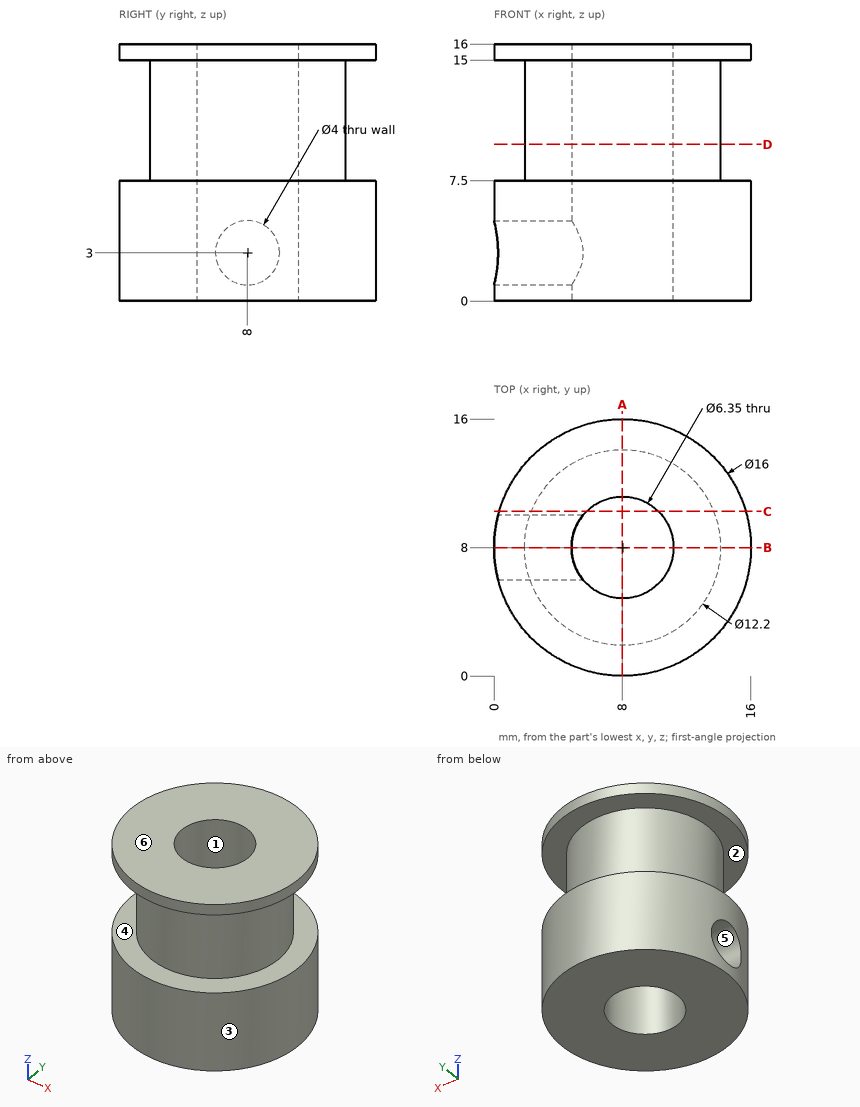
For this review, use the dimensioned drawing (mm, ordinates from the lowest corner) and the shaded views. A direction names the side the tool comes from. Coordinates: 2 decimals unless noted, no trailing zeros. Order: outer loops, then holes, each group sorted by start corner. A loop starts at its lowest first (then second) coordinate and runs counter-clockwise, first axis right, second up. Notation, with made-up numbers: (22.25, 29.25) - (33.25, 29.25) arc R19 cw to (33.25, 58.25) - close; hole circle Ø3 at (-21.5, 46.25). An arc over 180 degrees is marked (long way). Answer as a JSON object with one key per item and string values. Group by question number.
1. Clearance check with flat-ended pins moving along their axes: P1, Ø2, axis at x = 12.5, z = 9, coming from the +Y side; P2, Ø1.5, axis at x = 6, z = 5, coming from the -Y side; P3, Ø1.5, axis at y = 10.5, z = 12, coming from the -X side. State where each tip first meets the part, or that it passes through.
2. We need section D-D on z = 9.75. State the section outline as (x, y) points (3 decimals).
3. We need section A-A on x = 8. State the section outline as (y, z) points (3 decimals).
4. The part is to be moulded in two halves that separate along X. For the marked faces 1, 2 and 3, say which applies: pulls with the +X half, pulls with the -X half, needs draft (parallel to the pull), parting line crosses it, or undercut.
5. We need section B-B on y = 8. State the section outline as (x, z) points (3 decimals).
6. For probe 1 along Z at (x, y) = (14.5, 5.25); probe 2 along Y at (x, z) = (8, 4) (3 decimals); probe 3 along Y at (x, z) = (8, 10.75) (3 decimals), list the stretches that pass through material, from the lowest coordinate up.
7. For the marked faces 4, 5 and 6, list the 3-axis set-ups (+Z, -Z, +X, -X, +Y, -Y) from which the entire face can be reached by the end or side of a thin tool; tool diameter is ignored.
8. We need section C-C on y = 10.25. State the section outline as (x, z) points, then the cut area to 3 significant figures.
Final values:
{
 "1": {"P1": "y = 13", "P2": "y = 0.1", "P3": "x = 2.16"},
 "2": {"outline": "circle Ø12.2 at (8, 8); hole circle Ø6.35 at (8, 8)"},
 "3": {"outline": "(0, 0) - (4.825, 0) - (4.825, 16) - (0, 16) - (0, 15) - (1.9, 15) - (1.9, 7.5) - (0, 7.5) - close; (11.175, 0) - (16, 0) - (16, 7.5) - (14.1, 7.5) - (14.1, 15) - (16, 15) - (16, 16) - (11.175, 16) - close"},
 "4": {"face 1": "undercut", "face 2": "needs draft", "face 3": "parting line crosses it"},
 "5": {"outline": "(0, 0) - (4.825, 0) - (4.825, 1) - (0, 1) - close; (0, 5) - (4.825, 5) - (4.825, 16) - (0, 16) - (0, 15) - (1.9, 15) - (1.9, 7.5) - (0, 7.5) - close; (11.175, 0) - (16, 0) - (16, 7.5) - (14.1, 7.5) - (14.1, 15) - (16, 15) - (16, 16) - (11.175, 16) - close"},
 "6": {"probe 1": "0 to 7.5, 15 to 16", "probe 2": "0 to 4.825, 11.175 to 16", "probe 3": "1.9 to 4.825, 11.175 to 14.1"},
 "7": {"face 4": "none", "face 5": "-X", "face 6": "+Z, +X, -X, +Y, -Y"},
 "8": {"outline": "(0.32, 0) - (5.76, 0) - (5.76, 16) - (0.32, 16) - (0.32, 15) - (2.33, 15) - (2.33, 7.5) - (0.32, 7.5) - close; (10.24, 0) - (15.68, 0) - (15.68, 7.5) - (13.67, 7.5) - (13.67, 15) - (15.68, 15) - (15.68, 16) - (10.24, 16) - close", "area": "144 mm²"}
}
